Design review of the part shown in the three views and the two pictorial views. Dimensions are in mm from the part's minimum x, y and z. Round coordinates to 2 decimals unless told otherwise and drop trailing zeros. Loops run counter-clockwise (first coordinate to the right, second up) from the corner with the lowest first, then second, coordinate; pieces in that order, holes last.
1) Take a section at C-C (x = 10.5). State the section outline as (y, z) points (1 decimal).
2) Insertion check: pin 1 (1 mm diameter, centred on y = 1, z = 20.5, fed in from +X); pin 2 (1 mm diameter, centred on y = 1, z = 71, fed in from -X); pin 3 (4 mm diameter, centred on x = 51, z = 35, fed in from -Y). Each pin has a flat end and moves straight along its axis. Give the tip position at first contact, or say it passes through.
3) Take a section at A-A (y = 2.05). Give the number of separate pieces and of enclosed holes in the cut face.
4) Wall thickness on L1, parallel to X at y = 0.75, z = 51; L2, parallel to X at y = 1.4, z = 11 (1 decimal); L3, parallel to Z at x = 10, y = 2.2 (1 decimal): over which ranges is each line inside the solid? List them lowest first.
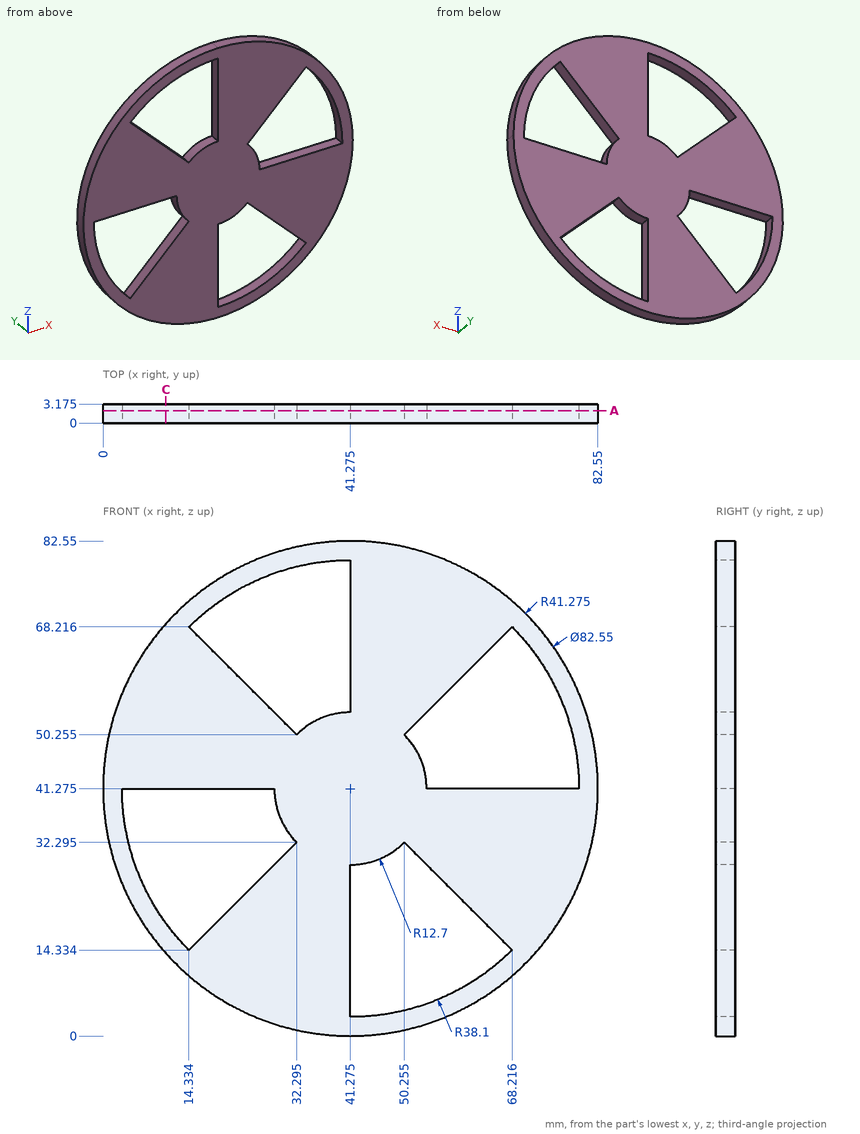
Response:
1. outline: (0, 13.8) - (3.2, 13.8) - (3.2, 18.8) - (0, 18.8) - close; (0, 41.3) - (3.2, 41.3) - (3.2, 68.8) - (0, 68.8) - close
2. pin 1: stops at x = 77.23
2. pin 2: stops at x = 12.13
2. pin 3: stops at y = 0
3. separate pieces: 1
3. enclosed holes: 4
4. L1: x = 1.16 to 31.55, 33.11 to 51, 78.11 to 81.39
4. L2: x = 13.2 to 41.3, 64.4 to 69.3
4. L3: z = 14.3 to 19.5, 41.3 to 68.2
